Autodesk Inventor part; units mm, degrees
ref_plane "YZ Plane" through (0, 0, 0) normal (1, 0, 0) x (0, 1, 0)
ref_plane "XZ Plane" through (0, 0, 0) normal (0, 1, 0) x (-1, 0, 0)
ref_plane "XY Plane" through (0, 0, 0) normal (0, 0, 1) x (1, 0, 0)
sketch "Sketch1" plane through (0, 0, 0) normal (0, 1, 0) x (-1, 0, 0)
  line L0 (-12.7, -12.7) -> (12.7, -12.7)
  line L1 (12.7, -12.7) -> (12.7, 12.7)
  line L2 (12.7, 12.7) -> (-12.7, 12.7)
  line L3 (-12.7, 12.7) -> (-12.7, -12.7)
  line L4 (-12.7, -12.7) -> (12.7, 12.7) construction
  line L5 (12.7, -12.7) -> (-12.7, 12.7) construction
  line L6 (9.525, 9.525) -> (9.525, -9.525)
  line L7 (9.525, -9.525) -> (-9.525, -9.525)
  line L8 (-9.525, -9.525) -> (-9.525, 9.525)
  line L9 (-9.525, 9.525) -> (9.525, 9.525)
  point P0 (0, 0)
  dimension "d0" = 25.4
  dimension "d1" = 25.4
  dimension "d2" = 3.175
extrude "Extrusion1" add sketch "Sketch1" along normal blind 323.3735
sketch "Sketch2" plane through (-12.7, 0, 12.7) normal (0, 0, 1) x (1, 0, 0)
  line L0 (0, 0) -> (25.4, 0)
  line L1 (25.4, 0) -> (25.4, 323.3735)
  line L2 (0, 323.3735) -> (25.4, 323.3735)
  line L3 (0, 0) -> (0, 323.3735)
  line L4 (163.521, 219.9589) -> (12.7, 323.3735)
  line L5 (12.7, 323.3735) -> (-138.121, 103.4146)
  line L6 (-138.121, 103.4146) -> (12.7, 0)
  line L7 (12.7, 0) -> (163.521, 219.9589)
  point P0 (0, 8.7081)
  point P1 (25.4, 18.5218)
  point P2 (0, 304.8517)
  point P3 (25.4, 314.6654)
  dimension "d5" = 266.7
extrude "Extrusion2" cut sketch "Sketch2" against normal through all contours L3 L6 L0 | L7 L1 L0 | L3 L2 L5 | L4 L2 L1
properties part number "STRU_014_BilletCrossbar3_Angled" material "Aluminum 6061"
Check sheet for the modelled part. Datum: model origin and axes. Units: mm. A direction names the side the tool comes from. Coordinates: 2 decimals unless noted, no trailing zeros. Write each loop counter-clockwise with the first axis right and the second up, starting at its lowest first coordinate (ties: lowest second). Pieces come first, ordered by that corner, then holes.
Item 1: Cross-section at B-B on y = 249. Record the boundary of the cut face in (x, z) (3 decimals).
Numbers:
outline: (-12.7, -12.7) - (12.7, -12.7) - (12.7, 12.7) - (-12.7, 12.7) - close; hole (-9.525, -9.525) - (9.525, -9.525) - (9.525, 9.525) - (-9.525, 9.525) - close
Item 2: Mould release check, pull along Z, two halves, no side actions. Record for faces 3 (the face through (0, 159, -9.525)), 4 (the face through (0, 159, 12.7)), 5 (the face through (0, 159, -12.7)), 6 (the face through (-12.7, 155, 0)): released by +Z, released by -Z, zero draft, split by the parting line, or undercut.
Numbers:
face 3: undercut
face 4: released by +Z
face 5: released by -Z
face 6: zero draft
Item 3: Access from +Z, -Z, +X, -X, +Y, -Y to the whole of each face (thin tool, end or side, straight path). Record for faces 1 (the face through (10.494, 15.305, 0.178)), 2 (the face through (0, 159, 9.525)).
Numbers:
face 1: +Z, -Z, +X, -Y
face 2: +Y, -Y
Item 4: Cross-section at A-A on z = -5. Record the boundary of the cut face in (x, y) (3 decimals).
Numbers:
outline: (-12.7, 8.708) - (-9.525, 6.531) - (-9.525, 309.482) - (-12.7, 304.852) - close; (9.525, 13.891) - (12.7, 18.522) - (12.7, 314.665) - (9.525, 316.842) - close
Item 5: Scan lines: probe 1 along Z at (x, y) = (0.25, 160.5) (3 decimals); probe 2 along Y at (x, z) = (-11.25, 5.5). Record each from-to range of solid material in increasing order.
Numbers:
probe 1: z = -12.7 to -9.525, 9.525 to 12.7
probe 2: y = 7.71 to 306.97
Item 6: Cross-section at C-C on x = 2.75. Record the boundary of the cut face in (y, z) (3 decimals).
Numbers:
outline: (4.011, -12.7) - (321.488, -12.7) - (321.488, -9.525) - (4.011, -9.525) - close; (4.011, 9.525) - (321.488, 9.525) - (321.488, 12.7) - (4.011, 12.7) - close
